```python
from build123d import *

# Parameters (mm, degrees)
F0_W     = 350
F0_H     = 200
F0_R     = 7.5
F1_DEPTH = 10
F2_R     = 87


with BuildPart() as f1:
    # F0 (on Front) → F1 (new body)
    with BuildSketch(Plane.XZ):
        Rectangle(F0_W, F0_H)
        with Locations((-58.5, 10)):
            Circle(F0_R, mode=Mode.SUBTRACT)
        with Locations((17.5, 10)):
            Circle(F0_R, mode=Mode.SUBTRACT)
        with Locations((70, 10)):
            Circle(F0_R, mode=Mode.SUBTRACT)
    extrude(amount=F1_DEPTH)

    # F2
    f2_edges = [f1.edges().sort_by_distance(p)[0] for p in [
        (175, -5, 100),
        (-175, -5, 100),
        (-175, -5, -100),
        (175, -5, -100),
    ]]
    fillet(f2_edges, radius=F2_R)


solid = f1.part
```
Verification items for the finished model (mm, model axes). Give positions to 0.01 mm unless a question says otherwise; leave off trailing zeros. Order: outer loops, then holes, each group sorted by start corner. A loop starts at its lowest first (then second) coordinate and runs counter-clockwise, first axis right, second up. Notation, with made-up numbers: (82.25, -20.75) - (112.25, -20.75) arc R27 cw to (112.25, 13.25) - close; hole circle Ø11 at (67.5, -1). An arc over 180 degrees is marked (long way). Answer as CSV lines item,"result". Start each with the question number.
Item 1: Section check B-B, the plane x = -58.5. Record the boundary of the cut face in (y, z), plus the area to 3 significant figures.
Item 2: Gauge pin test, flat ends, axial feed: pin 1 (3 mm diameter, centred on y = -6.5, z = 57.5, fed in from +X); pin 2 (4 mm diameter, centred on y = -5.5, z = -54.5, fed in from +X); pin 3 (3 mm diameter, centred on y = -3, z = -30.5, fed in from +X). Record the tip position at first contact, or that the pin passes through.
Item 3: Section check C-C, the plane z = 54. Record the boundary of the cut face in (x, y).
Item 4: Section check A-A, the plane y = -7. Record the boundary of the cut face in (x, z).
Item 5: Material ranges on L1, parallel to Z at x = 70, y = -2.25; L2, parallel to X at y = -6, z = -26; L3, parallel to X at y = -1, z = -60.5, recorded low to high.
Item 6: Mould release check, pull along X, two halves, no side actions. Record for faces 1 (the face through (-150.19, -5.07, -73.84)), 2 (the face through (148.84, -5.07, -75.19)), 3 (the face through (62.507, -4.93, 10.33)), 4 (the face through (-64.452, -4.93, 5.436)): released by +X, released by -X, zero draft, split by the parting line, or undercut.
Filled in:
1,outline,"(-10, -100) - (0, -100) - (0, 2.5) - (-10, 2.5) - close; (-10, 17.5) - (0, 17.5) - (0, 100) - (-10, 100) - close"
1,area,"1,850 mm^2"
2,pin 1,"x = 163.63"
2,pin 2,"x = 165.52"
2,pin 3,"x = 173.52"
3,outline,"(-164.73, -10) - (164.73, -10) - (164.73, 0) - (-164.73, 0) - close"
4,outline,"(-175, -13) arc R87 ccw to (-88, -100) - (88, -100) arc R87 ccw to (175, -13) - (175, 13) arc R87 ccw to (88, 100) - (-88, 100) arc R87 ccw to (-175, 13) - close; hole circle Ø15 at (-58.5, 10); hole circle Ø15 at (17.5, 10); hole circle Ø15 at (70, 10)"
5,L1,"-100 to 2.5, 17.5 to 100"
5,L2,"-174.02 to 174.02"
5,L3,"-160.89 to 160.89"
6,face 1,"released by -X"
6,face 2,"released by +X"
6,face 3,"undercut"
6,face 4,"undercut"
